Part model, mm, in its own coordinate system. Round coordinates to 2 decimals unless told otherwise and drop trailing zeros. Order: outer loops, then holes, each group sorted by start corner. A loop starts at its lowest first (then second) coordinate and runs counter-clockwise, first axis right, second up. Notation, with made-up numbers: (37, 80) -> (83, 80) arc R22 ccw to (83, 92) -> close; hole circle Ø4 at (-17, 62.25). An arc over 180 degrees is marked (long way). Return JSON: item names as keys, results as strings. Group by question number.
from build123d import *

# Parameters (mm, degrees)
SKETCH2_W           = 30
SKETCH2_H           = 10
BOSS_EXTRUDE1_DEPTH = 250
SKETCH3_R           = 6
CUT_EXTRUDE1_DEPTH  = 30
FILLET1_R           = 10
FILLET3_R           = 10
CUT_EXTRUDE2_START  = -40
CUT_EXTRUDE2_DEPTH  = 40
FILLET4_R           = 5
FILLET5_R           = 5
FILLET6_R           = 5


with BuildPart() as part:
    # Sketch2 → Boss-Extrude1 (new body)
    with BuildSketch(Plane.XY):
        with Locations((15, 5)):
            Rectangle(SKETCH2_W, SKETCH2_H)
    extrude(amount=BOSS_EXTRUDE1_DEPTH)

    # Sketch3 → Cut-Extrude1 (cut)
    with BuildSketch(Plane(origin=(0, 10, 0), x_dir=(1, 0, 0), z_dir=(0, 1, 0))):
        with Locations(Location((15, -7, 0), (0, 0, 270))):
            Circle(SKETCH3_R)
    extrude(amount=-CUT_EXTRUDE1_DEPTH, mode=Mode.SUBTRACT)

    # Fillet1
    fillet1_edges = [part.edges().sort_by_distance(p)[0] for p in [
        (30, 5, 0),
    ]]
    fillet(fillet1_edges, radius=FILLET1_R)

    # Fillet3
    fillet3_edges = [part.edges().sort_by_distance(p)[0] for p in [
        (0, 5, 0),
    ]]
    fillet(fillet3_edges, radius=FILLET3_R)

    # Cut-Extrude2: read off the stored shape, not the designer's step
    # Cut-Extrude2 outline → Cut-Extrude2 (cut)
    with BuildSketch(Plane.XY.offset(250).offset(CUT_EXTRUDE2_START)):
        with BuildLine():
            Line((4, 5.122217373), (4.687433408, 5.134216568))
            ThreePointArc((4.687433408, 5.134216568), (5.779010382, 5.481326474), (6.501094127, 6.370494985))
            Line((6.501094127, 6.370494985), (8, 10))
            Line((8, 10), (0, 10))
            Line((0, 10), (0, 5))
            Line((0, 5), (1, 5.017455065))
            Line((1, 5.017455065), (4, 5.122217373))
        make_face()
        with BuildLine():
            Line((1, 4.982544935), (0, 5))
            Line((0, 5), (0, 0))
            Line((0, 0), (8, 0))
            Line((8, 0), (6.501094127, 3.629505015))
            ThreePointArc((6.501094127, 3.629505015), (5.779010382, 4.518673526), (4.687433408, 4.865783432))
            Line((4.687433408, 4.865783432), (4, 4.877782627))
            Line((4, 4.877782627), (1, 4.982544935))
        make_face()
    extrude(amount=CUT_EXTRUDE2_DEPTH, mode=Mode.SUBTRACT)

    # Fillet4
    fillet4_edges = [part.edges().sort_by_distance(p)[0] for p in [
        (8, 10, 230),
    ]]
    fillet(fillet4_edges, radius=FILLET4_R)

    # Fillet5
    fillet5_edges = [part.edges().sort_by_distance(p)[0] for p in [
        (8, 0, 230),
    ]]
    fillet(fillet5_edges, radius=FILLET5_R)

    # Fillet6
    fillet6_edges = [part.edges().sort_by_distance(p)[0] for p in [
        (30, 5, 250),
    ]]
    fillet(fillet6_edges, radius=FILLET6_R)


solid = part.part
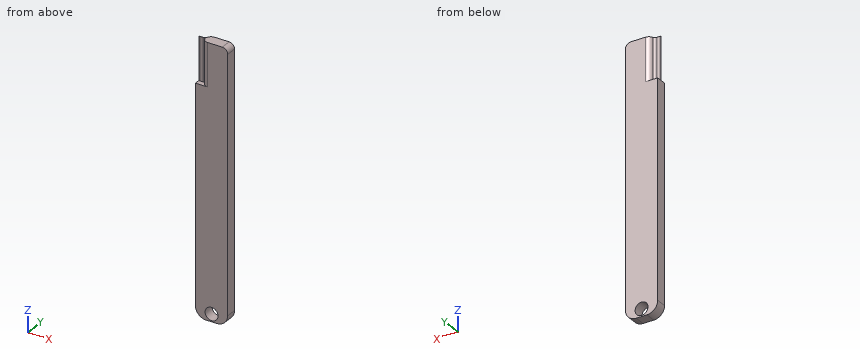
(1) Saw through at C-C, the plane z = 7. List the corners of the cut face in (x, y).
(2) Saw through at B-B, the plane y = 8.5. List the corners of the cut face in (x, z), and give its area (3 significant figures).
(3) Probe L1, parallel to X at y = 6.5, z = 7; L2, parallel to Z at x = 16, y = 9.75; L3, parallel to Z at x = 12, y = 8.75. List the from-to ranges inside material, lowest first. Write a range as [from, to].
(4) Saw through at A-A, the plane x = 15. List the corners of the cut face in (y, z), and give its area (3 significant figures).
Results are:
{
 "1": {"outline": "(0.46, 0) -> (9, 0) -> (9, 10) -> (0.46, 10) -> close; (21, 0) -> (29.54, 0) -> (29.54, 10) -> (21, 10) -> close"},
 "2": {"outline": "(0, 10) arc R10 ccw to (10, 0) -> (20, 0) arc R10 ccw to (30, 10) -> (30, 245) arc R5 ccw to (25, 250) -> (7.77, 250) -> (7.77, 210) -> (0, 210) -> close; hole circle Ø12 at (15, 7)", "area": "7,030 mm^2"},
 "3": {"L1": "x = [0.46, 9], [21, 29.54]", "L2": "z = [0, 1.08], [12.92, 250]", "L3": "z = [0, 1.8], [12.2, 250]"},
 "4": {"outline": "(0, 0) -> (10, 0) -> (10, 1) -> (0, 1) -> close; (0, 13) -> (10, 13) -> (10, 250) -> (0, 250) -> close", "area": "2,380 mm^2"}
}
